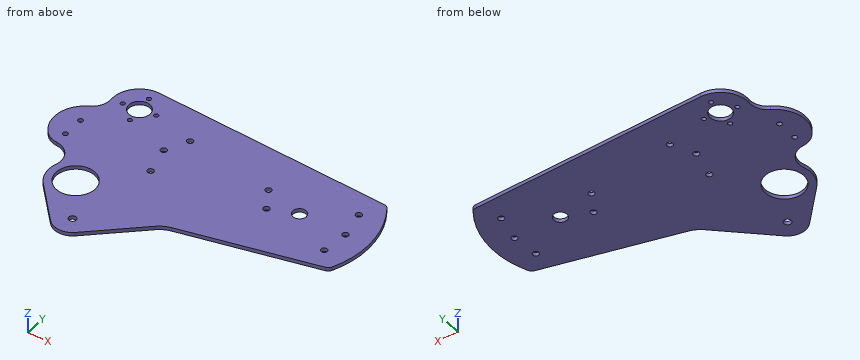
```python
from build123d import *

# Parameters (mm, degrees)
SKETCH1_R           = 3
SKETCH1_R_2         = 2
SKETCH1_R_3         = 2.5
SKETCH1_R_4         = 1.75
SKETCH1_R_5         = 8.75
SKETCH1_R_6         = 5.5
SKETCH1_R_7         = 16
BOSS_EXTRUDE1_DEPTH = 3


with BuildPart() as part:
    # Sketch1 → Boss-Extrude1 (new body)
    with BuildSketch(Plane.XY):
        with BuildLine():
            ThreePointArc((-111.886028634, 49.480245878), (-128.824449864, 42.592956949), (-134.705774542, 25.279526249))
            ThreePointArc((-134.705774542, 25.279526249), (-136.343375771, 16.802270376), (-142.382746132, 10.632050724))
            ThreePointArc((-142.382746132, 10.632050724), (-155.099864059, -8.058287742), (-147.542861296, -29.364285714))
            ThreePointArc((-147.542861296, -29.364285714), (-143.125485566, -32.280163581), (-137.970351553, -33.480224156))
            ThreePointArc((-137.970351553, -33.480224156), (-126.431132561, -39.888203569), (-124.422839539, -52.93360637))
            ThreePointArc((-124.422839539, -52.93360637), (-124.888175134, -64.31939994), (-119.594822483, -74.410646153))
            Line((-119.594822483, -74.410646153), (-92.540517723, -103.740413224))
            ThreePointArc((-92.540517723, -103.740413224), (-82.119700521, -108.557935129), (-71.344567605, -104.595807028))
            Line((-71.344567605, -104.595807028), (-31.441449774, -67.788453323))
            ThreePointArc((-31.441449774, -67.788453323), (-26.802171393, -64.493076397), (-21.481893225, -62.473904985))
            Line((-21.481893225, -62.473904985), (87.599861039, -36.324111832))
            ThreePointArc((87.599861039, -36.324111832), (89.628937626, -35.308169791), (91, -33.5))
            ThreePointArc((91, -33.5), (97.203558128, 3.661751943), (84.51565505, 39.137054004))
            ThreePointArc((84.51565505, 39.137054004), (82.813644384, 40.69192784), (80.594954641, 41.317938046))
            Line((80.594954641, 41.317938046), (-111.886028634, 49.480245878))
        make_face()
        with Locations((-81.514845762, -93.570135067)):
            Circle(SKETCH1_R, mode=Mode.SUBTRACT)
        with Locations((-138.3, -22.75)):
            Circle(SKETCH1_R_2, mode=Mode.SUBTRACT)
        with Locations((-138.3, -5.25)):
            Circle(SKETCH1_R_2, mode=Mode.SUBTRACT)
        with Locations((-68.3, -21.5)):
            Circle(SKETCH1_R_3, mode=Mode.SUBTRACT)
        with Locations((-74.1, 1.7)):
            Circle(SKETCH1_R_3, mode=Mode.SUBTRACT)
        with Locations((-111.422396488, 14.575141755)):
            Circle(SKETCH1_R_4, mode=Mode.SUBTRACT)
        with Locations((-125.742976533, 26.1042782)):
            Circle(SKETCH1_R_4, mode=Mode.SUBTRACT)
        with Locations((-112.818118288, 27.5)):
            Circle(SKETCH1_R_5, mode=Mode.SUBTRACT)
        with Locations((-114.213840088, 40.424858245)):
            Circle(SKETCH1_R_4, mode=Mode.SUBTRACT)
        with Locations((-99.893260043, 28.8957218)):
            Circle(SKETCH1_R_4, mode=Mode.SUBTRACT)
        with Locations((-65.3, 20)):
            Circle(SKETCH1_R_3, mode=Mode.SUBTRACT)
        with Locations((18.7, -8.7)):
            Circle(SKETCH1_R_3, mode=Mode.SUBTRACT)
        with Locations((76.2, -22)):
            Circle(SKETCH1_R_3, mode=Mode.SUBTRACT)
        with Locations((40.017782272, 0)):
            Circle(SKETCH1_R_6, mode=Mode.SUBTRACT)
        with Locations((78.2, -0.1)):
            Circle(SKETCH1_R_3, mode=Mode.SUBTRACT)
        with Locations((8.2, 8.3)):
            Circle(SKETCH1_R_3, mode=Mode.SUBTRACT)
        with Locations((73.2, 22.3)):
            Circle(SKETCH1_R_3, mode=Mode.SUBTRACT)
        with Locations((-103.42383694, -59.494238188)):
            Circle(SKETCH1_R_7, mode=Mode.SUBTRACT)
    extrude(amount=BOSS_EXTRUDE1_DEPTH)


solid = part.part
```
Build history of the part. All positions in model axes, mm. Give positions to 0.01 mm unless a question says otherwise; leave off trailing zeros. Loops run counter-clockwise (first coordinate to the right, second up) from the corner with the lowest first, then second, coordinate; pieces in that order, holes last.
Item 1: Slice it at C-C, the plane x = -18.5. List the corners of the cut face in (y, z), and give its area (3 significant figures).
Answers follow:
outline: (-61.76, 0) - (45.52, 0) - (45.52, 3) - (-61.76, 3) - close
area: 322 mm2
Item 2: Slice it at A-A, the plane z = 0.55. Give the number of separate pieces and of enclosed holes in the cut face, and give its area (3 significant figures).
Answers follow:
separate pieces: 1
enclosed holes: 18
area: 24,800 mm2
Item 3: Slice it at B-B, the plane x = 18.7. List the corners of the cut face in (y, z).
Answers follow:
outline: (-52.84, 0) - (-11.2, 0) - (-11.2, 3) - (-52.84, 3) - close; (-6.2, 0) - (43.94, 0) - (43.94, 3) - (-6.2, 3) - close
Item 4: Flat gauge pins, fed straight in: pin 1 (3 mm diameter, centred on x = -125.74, y = 26.1, fed in from -Z); pin 2 (1 mm diameter, centred on x = 24, z = 1, fed in from -Y); pin 3 (1.5 mm diameter, centred on x = -41.5, z = 1.5, fed in from +Y); pin 4 (1 mm diameter, centred on y = -60, z = 2, fed in from -X). Where does each tip first touch, or does it go through?
Answers follow:
pin 1: passes through
pin 2: stops at y = -51.69
pin 3: stops at y = 46.53
pin 4: stops at x = -125.42
Item 5: Drill centre lines: line 1 (Y direction, x = -140, z = 2.35); line 2 (X direction, y = -23, z = 0.3); line 3 (Y direction, x = 76.2, z = 1.7). Where is each one in solid material? Low to high.
Answers follow:
line 1: y = -33.24 to -23.8, -21.7 to -6.3, -4.2 to 12.26
line 2: x = -152.38 to -140.28, -136.32 to -70.3, -66.3 to 73.91, 78.49 to 94.78
line 3: y = -39.06 to -24.5, -19.5 to -1.6, 1.4 to 41.5
Item 6: Slice it at D-D, the plane x = -45. List the corners of the cut face in (y, z).
Answers follow:
outline: (-80.3, 0) - (46.64, 0) - (46.64, 3) - (-80.3, 3) - close
